from build123d import *

# Parameters (mm, degrees)
SKETCH1_R                   = 9.5
BOSS_EXTRUDE1_DEPTH         = 20
SKETCH2_R                   = 7.5
BOSS_EXTRUDE2_DEPTH         = 58
SKETCH3_R                   = 6
BOSS_EXTRUDE3_DEPTH         = 18
BOSS_EXTRUDE4_START         = 21
SKETCH4_R                   = 7.5
BOSS_EXTRUDE4_DEPTH         = 21
CUT_EXTRUDE1_DEPTH          = 2
TAP_DRILL_FOR_M4_TAP1_D     = 5
TAP_DRILL_FOR_M4_TAP1_DEPTH = 10
TAP_DRILL_FOR_M4_TAP1_TIP   = 1.502151548
CHAMFER1_SIZE               = 1
CHAMFER2_SIZE               = 3


with BuildPart() as part:
    # Sketch1 → Boss-Extrude1 (new body)
    with BuildSketch(Plane(origin=(0, 0, 0), x_dir=(-1, 0, 0), z_dir=(0, 1, 0))):
        with Locations(Location((0, 0, 0), (0, 0, 90))):
            Circle(SKETCH1_R)
    extrude(amount=BOSS_EXTRUDE1_DEPTH)

    # Sketch2 → Boss-Extrude2 (add)
    with BuildSketch(Plane.XZ):
        with Locations(Location((0, -2, 0), (0, 0, 270))):
            Circle(SKETCH2_R)
    extrude(amount=BOSS_EXTRUDE2_DEPTH)

    # Sketch3 → Boss-Extrude3 (add)
    with BuildSketch(Plane.XZ.offset(58)):
        with Locations(Location((0, -2, 0), (0, 0, 270))):
            Circle(SKETCH3_R)
    extrude(amount=BOSS_EXTRUDE3_DEPTH)

    # Sketch4 → Boss-Extrude4 (add)
    with BuildSketch(Plane(origin=(0, 20, 0), x_dir=(-1, 0, 0), z_dir=(0, 1, 0)).offset(BOSS_EXTRUDE4_START)):
        with Locations(Location((0, -2, 0), (0, 0, 270))):
            Circle(SKETCH4_R)
    extrude(amount=-BOSS_EXTRUDE4_DEPTH)

    # Sketch5 → Cut-Extrude1 (cut)
    with BuildSketch(Plane(origin=(0, 0, 4), x_dir=(0, 1, 0), z_dir=(0, 0, 1))):
        with BuildLine():
            Line((-71, 2), (-61, 2))
            ThreePointArc((-61, 2), (-59, 0), (-61, -2))
            Line((-61, -2), (-71, -2))
            ThreePointArc((-71, -2), (-73, 0), (-71, 2))
        make_face()
    extrude(amount=-CUT_EXTRUDE1_DEPTH, mode=Mode.SUBTRACT)

    # Tap Drill for M4 Tap1
    with Locations(Plane.XZ.offset(76)):
        with Locations((0, -2)):
            Hole(TAP_DRILL_FOR_M4_TAP1_D / 2, depth=TAP_DRILL_FOR_M4_TAP1_DEPTH)
            with Locations((0, 0, -(TAP_DRILL_FOR_M4_TAP1_DEPTH + TAP_DRILL_FOR_M4_TAP1_TIP / 2))):  # 118° drill point
                Cone(0, TAP_DRILL_FOR_M4_TAP1_D / 2, TAP_DRILL_FOR_M4_TAP1_TIP, mode=Mode.SUBTRACT)

    # Chamfer1
    chamfer1_edges = [part.edges().sort_by_distance(p)[0] for p in [
        (0, 41, 5.5),
    ]]
    chamfer(chamfer1_edges, length=CHAMFER1_SIZE)

    # Chamfer2
    # the kernel refuses this chamfer: 3 mm, written as the material it takes off along each edge
    with BuildSketch(Plane(origin=(0, -58, -2), x_dir=(0, 0, -1), z_dir=(-1, 0, 0))) as chamfer2_piece_1_section:
        Polygon((7.5, -CHAMFER2_SIZE), (7.5 - CHAMFER2_SIZE, 0), (7.5, 0), align=None)
    chamfer2_piece_1 = revolve(axis=Axis((0, -58, -2), (0, -1, 0)), mode=Mode.PRIVATE)
    chamfer2_piece_1 = chamfer2_piece_1 - Plane(origin=(0, -55.74588243, -2), x_dir=(0, 0, -1), z_dir=(0, 1, 0)) * Cylinder(6, 30, mode=Mode.PRIVATE)
    add(chamfer2_piece_1, mode=Mode.SUBTRACT)


solid = part.part
The model under review builds one solid part; all positions refer to its coordinate system, in mm. A direction names the side the tool comes from. Coordinates: 2 decimals unless noted, no trailing zeros. Loops run counter-clockwise (first coordinate to the right, second up) from the corner with the lowest first, then second, coordinate; pieces in that order, holes last. Notation, with made-up numbers: (22.25, -23) -> (44.25, -23) arc R16 ccw to (44.25, -17) -> close; hole circle Ø9 at (-27.5, 46). An arc over 180 degrees is marked (long way). Use a Markdown table: item, result. Add a question column.
1. Clearance check with flat-ended pins moving along their axes: pin 1 Ø1 at (x, y) = (-1.5, -45.5) entering from +Z; pin 2 Ø8 at (x, z) = (-0.5, -0.5) entering from -Y; pin 3 Ø1.8 at (y, z) = (-64, 3) entering from +X; pin 4 Ø5 at (y, z) = (-59.5, 1) entering from +X. State where each tip first meets the part, or that it passes through.
2. Draft analysis for pull direction Z (two halves, no side actions). For faces 5 (the face through (0, 0, 6)), 6 (the face through (-0.094, -64.759, -2.424)), 7 (the face through (-1.15, -70.93, -4.22)), 8 (the face through (0, -66, 2)), state which applies: pulls with the +Z half, pulls with the -Z half, needs draft (parallel to the pull), parting line crosses it, or undercut.
3. To check wall thickness, follow line 1 (Z direction, x = 0, y = -69.5); line 2 (Z direction, x = 0, y = -74); line 3 (X direction, y = -70.75, z = -2). State the ranges of each line that lie inside material, in increasing order.
4. Add section A-A on y = 27. Write out the cut boundary in (x, z).
5. Machinability: for faces 1 (the face through (-0.33, 30.14, 5.493)), 2 (the face through (0, -59, 3)), 3 (the face through (0, -76, -5)), 4 (the face through (0.33, -27.115, 5.493)), which of the approach directions +Z, -Z, +X, -X, +Y, -Y give a long, thin tool a straight path to every point of the face, cutting with its end or side? Answer none if there is none.
Returned:
| question | item | result |
|---|---|---|
| 1 | pin 1 | stops at z = 5.43 |
| 1 | pin 2 | stops at y = -76 |
| 1 | pin 3 | stops at x = 4.38 |
| 1 | pin 4 | stops at x = 5.98 |
| 2 | face 5 | needs draft |
| 2 | face 6 | undercut |
| 2 | face 7 | undercut |
| 2 | face 8 | pulls with the +Z half |
| 3 | line 1 | z = -8 to -4.5, 0.5 to 2 |
| 3 | line 2 | z = -8 to -4.5, 0.5 to 4 |
| 3 | line 3 | x = -6 to -2.5, 2.5 to 6 |
| 4 | outline | circle Ø15 at (0, -2) |
| 5 | face 1 | +Y |
| 5 | face 2 | +Z |
| 5 | face 3 | +Z, -Z, +X, -X, -Y |
| 5 | face 4 | -Y |
